Check sheet for the modelled part. Datum: model origin and axes. Units: mm. A direction names the side the tool comes from. Give positions to 0.01 mm unless a question says otherwise; leave off trailing zeros. Write each loop counter-clockwise with the first axis right and the second up, starting at its lowest first coordinate (ties: lowest second). Pieces come first, ordered by that corner, then holes. Notation, with made-up numbers: M 3.25,11.25 L 7.25,11.25 A14 cw 7.25,27.25 Z; hole C 2,-23 d4. An arc over 180 degrees is marked long. Use CSV: the item, a comma, the result in double quotes. Start each with the question number.
1. Cross-section at A-A, the plane z = 0. Enter the section's corners in (x, y), and give its area (3 significant figures).
2. Depth check by flat-ended pin: P1, Ø1.5, axis at x = -1, y = 39.5, coming from the +Z side; P2, Ø1.7, axis at y = 55, z = 0, coming from the -X side. Enter the tip coordinate at first touch or a pass-through.
3. Scan lines: line 1 (Y direction, x = -1.1, z = -0.75); line 2 (X direction, y = 28, z = 0.2); line 3 (Z direction, x = 0.85, y = 16). Record each from-to range of solid material in increasing order.
4. Access from +Z, -Z, +X, -X, +Y, -Y to the whole of each face (thin tool, end or side, straight path). Record for faces 4 (the face through (-1.4, 18.4, 0)), 5 (the face through (0, 0, 0)), 6 (the face through (-1, 56, 0)).
5. Cross-section at B-B, the plane y = 11. Enter the section's corners in (x, z).
6. Mould release check, pull along Y, two halves, no side actions. Record for faces 1 (the face through (-1.4, 24.4, 0)), 2 (the face through (1.6, 29.6, 1.2)), 3 (the face through (0, 60, 0)): +Y half, -Y half, draft (parallel to the pull), parting line (faces both ways), or undercut.
Autodesk Inventor part; units mm, degrees
ref_plane "作業平面1" through (0, 21.4, 0) normal (0, 1, 0) x (-1, 0, 0)
ref_plane "YZ Plane" through (0, 0, 0) normal (1, 0, 0) x (0, 1, 0)
ref_plane "XZ Plane" through (0, 0, 0) normal (0, 1, 0) x (-1, 0, 0)
sketch "スケッチ1" plane through (0, 0, 0) normal (0, 1, 0) x (-1, 0, 0)
  circle A0 centre (0, 0) radius 2
  dimension "d0" = 4
extrude "押し出し1" add sketch "スケッチ1" along normal blind 60
sketch "スケッチ2" plane through (0, 60, 0) normal (0, 1, 0) x (1, 0, 0)
  circle A0 centre (0, 0) radius 2
  line L0 (-1, -1.7321) -> (-1, 1.7321)
  dimension "d3" = 1
extrude "押し出し2" cut sketch "スケッチ2" against normal blind 7.8 contours L0 A0 picked at (-1.1242, -0.4849)
chamfer "面取り1" distance 0.2 angle 45 2 edges at (2, 60, 0) (2, 0, 0)
sketch "スケッチ3" plane through (0, 0, 0) normal (0, 0, 1) x (1, 0, 0)
  line L0 (-2, 18.4) -> (-1, 18.4)
  line L1 (-1, 18.4) -> (-1, 21.4)
  line L2 (-1, 21.4) -> (-2, 21.4)
  line L3 (-2, 21.4) -> (-2, 18.4)
  line L4 (1.8, 0) -> (-1.8, 0)
  line L5 (-2, 24.4) -> (-1, 24.4)
  line L6 (-1, 24.4) -> (-1, 21.4)
  line L7 (-2, 21.4) -> (-2, 24.4)
  line L8 (-2, 0.2) -> (-2, 52.2)
  point P0 (0, 0)
  dimension "d9" = 1
  dimension "d10" = 3
  dimension "d11" = 21.4
extrude "押し出し3" cut sketch "スケッチ3" along normal mid plane 55
ref_plane "作業平面1" through (0, 21.4, 0) normal (0, 1, 0) x (-1, 0, 0)
sketch "スケッチ5" plane through (0, 21.4, 0) normal (0, 1, 0) x (-1, 0, 0)
  line L0 (0, 0) -> (7.6217, 0)
properties part number "shaft" material "アルミニウム 6061"
Worked answers:
1,outline,"M -2,0.2 L -1.8,0 L 1.8,0 L 2,0.2 L 2,59.8 L 1.8,60 L -1,60 L -1,52.2 L -2,52.2 L -2,24.4 L -1,24.4 L -1,18.4 L -2,18.4 Z"
1,area,"226 mm^2"
2,P1,"stops at z = 1.98"
2,P2,"stops at x = -1"
3,line 1,"y = 0 to 18.4, 24.4 to 52.2"
3,line 2,"x = -1.99 to 1.99"
3,line 3,"z = -1.81 to 1.81"
4,face 4,"+Z, -Z, -X"
4,face 5,"+Z, -Z, +X, -X, -Y"
4,face 6,"+Z, -Z, -X, +Y"
5,outline,"C 0,0 d4"
6,face 1,"undercut"
6,face 2,"draft"
6,face 3,"+Y half"
